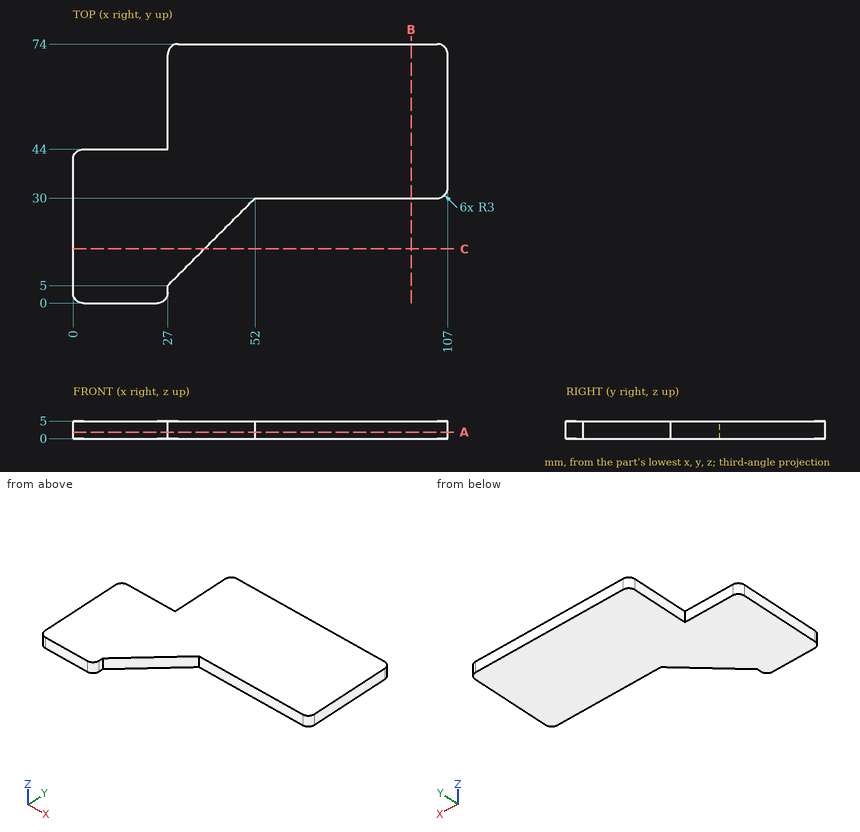
Study the drawing (mm; zero at the part's minimum x, y, z) and answer. Give positions to 0.01 mm unless a question says otherwise; leave off trailing zeros. Order: outer loops, then holes, each group sorted by start corner. A loop starts at its lowest first (then second) coordinate and runs counter-clockwise, first axis right, second up. Notation, with made-up numbers: M -21.75,-27.75 L 30.25,-27.75 A22 ccw 30.25,-15.75 Z; hole C 71.25,68.25 d6. An arc over 180 degrees is marked long. Put each result on its own line as item: value. Start each with the question number.
Item 1: Find the intervals of material crossed by line 1 along X through (y, z) = (66, 2.2); line 2 along Y through (x, z) = (98, 1.25); line 3 along Y through (x, z) = (20, 1.8), in increasing order.
Item 2: The part is cut by section A-A, the plane z = 1.85. Determine the outline of the cut face in (x, y).
Item 3: The part is cut by section B-B, the plane x = 96.5. Determine the outline of the cut face in (y, z), and give its area (3 significant figures).
Item 4: Flat-ended cylindrical pins translate along their axes: P1, Ø2, axis at y = 52.5, z = 2, coming from the -X side; P2, Ø12, axis at x = 58, y = 42.5, coming from the -Z side; P3, Ø1.5, axis at x = 77, z = 3.5, coming from the -Y side; P4, Ø1, axis at y = 4, z = 3.5, coming from the +X side. Find the tip coordinate at first contact, or state that the pin passes through.
Item 5: The part is cut by section C-C, the plane y = 15.5. Determine the outline of the cut face in (x, z).
Answer key:
1. line 1: x = 27 to 107
1. line 2: y = 30 to 74
1. line 3: y = 0 to 44
2. outline: M 0,3 A3 ccw 3,0 L 24,0 A3 ccw 27,3 L 27,5 L 52,30 L 104,30 A3 ccw 107,33 L 107,71 A3 ccw 104,74 L 30,74 A3 ccw 27,71 L 27,44 L 3,44 A3 ccw 0,41 Z
3. outline: M 30,0 L 74,0 L 74,5 L 30,5 Z
3. area: 220 mm²
4. P1: stops at x = 27
4. P2: stops at z = 0
4. P3: stops at y = 30
4. P4: stops at x = 27
5. outline: M 0,0 L 37.5,0 L 37.5,5 L 0,5 Z
